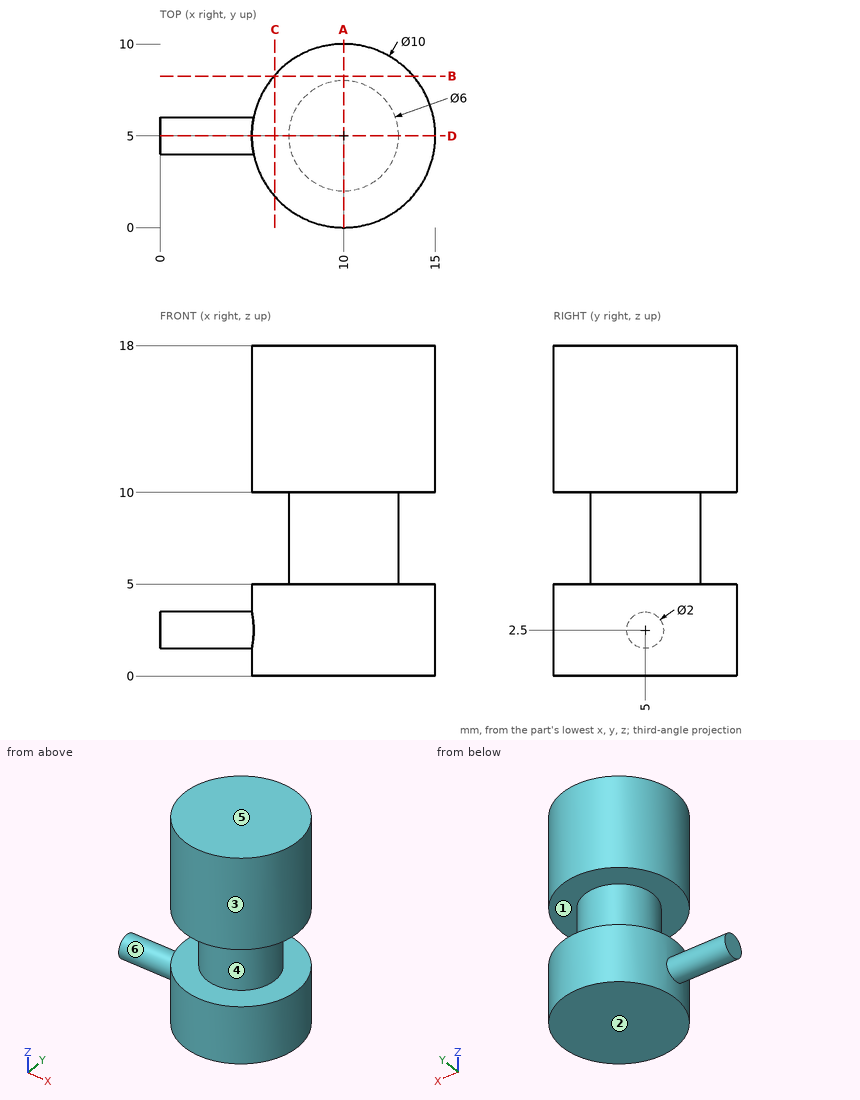
Print and shaded views of the part. All mm, measured from the part's lowest x, y and z. A direction names the side the tool comes from. Coordinates: 2 decimals unless noted, no trailing zeros. Loops run counter-clockwise (first coordinate to the right, second up) from the corner with the lowest first, then second, coordinate; pieces in that order, holes last. Notation, with made-up numbers: (-23.5, 45) - (15.5, 45) arc R31 cw to (15.5, 71) - close; hole circle Ø8 at (-36.75, 36.5). An arc over 180 degrees is marked (long way). Write item = value, one per line. Start each with the question number.
Item 1: 3-axis set-ups, long thin cutter, end or side, ignore diameter. For the marked faces 4, 5 and 6: which of +Z, -Z, +X, -X, +Y, -Y reach the whole face in a straight line?
Item 2: Drop flat-ended pins along their axis: pin 1 Ø6 at (y, z) = (4, 13) entering from -X; pin 2 Ø2 at (x, z) = (7, 7) entering from +Y; pin 3 Ø1 at (y, z) = (8, 2) entering from +X. Give the stop position or say it passes through.
Item 3: Saw through at C-C, the plane x = 6.25. List the corners of the cut face in (y, z).
Item 4: Pull direction Z, two halves, no side cores. Call the marked faces 1, 2 and 3: +Z half, -Z half, draft (parallel to the pull), parting line (faces both ways), or undercut.
Item 5: Saw through at D-D, the plane y = 5. List the corners of the cut face in (x, z).
Item 6: Saw through at A-A, the plane x = 10. List the corners of the cut face in (y, z), then the cut area to 3 significant figures.
Item 7: Wall check: probe 1 along Z at (x, y) = (10, 8.75); probe 2 along X at (y, z) = (9, 15.75); probe 3 along X at (y, z) = (7, 10.25). Give the ranges that are in metal, low to high. Write a range as [from, to].
Item 8: Saw through at B-B, the plane y = 8.25. List the corners of the cut face in (x, z).
Answers:
q1.face_4 = none
q1.face_5 = +Z, +X, -X, +Y, -Y
q1.face_6 = -X
q2.pin_1 = 5
q2.pin_2 = 7.24
q2.pin_3 = 14.33
q3.outline = (1.69, 0) - (8.31, 0) - (8.31, 5) - (1.69, 5) - close; (1.69, 10) - (8.31, 10) - (8.31, 18) - (1.69, 18) - close
q4.face_1 = undercut
q4.face_2 = -Z half
q4.face_3 = draft
q5.outline = (0, 1.5) - (5, 1.5) - (5, 0) - (15, 0) - (15, 5) - (13, 5) - (13, 10) - (15, 10) - (15, 18) - (5, 18) - (5, 10) - (7, 10) - (7, 5) - (5, 5) - (5, 3.5) - (0, 3.5) - close
q6.outline = (0, 0) - (10, 0) - (10, 5) - (8, 5) - (8, 10) - (10, 10) - (10, 18) - (0, 18) - (0, 10) - (2, 10) - (2, 5) - (0, 5) - close
q6.area = 160 mm2
q7.probe_1 = [0, 5], [10, 18]
q7.probe_2 = [7, 13]
q7.probe_3 = [5.42, 14.58]
q8.outline = (6.2, 0) - (13.8, 0) - (13.8, 5) - (6.2, 5) - close; (6.2, 10) - (13.8, 10) - (13.8, 18) - (6.2, 18) - close
